Build history of the part. All positions in model axes, mm. Coordinates: 2 decimals unless noted, no trailing zeros. Order: outer loops, then holes, each group sorted by start corner. A loop starts at its lowest first (then second) coordinate and runs counter-clockwise, first axis right, second up. Notation, with made-up numbers: (87, -25) - (115, -25) arc R21 cw to (115, 7) - close; hole circle Ø6 at (81, 32.25). An arc over 180 degrees is marked (long way). Answer as CSV lines item,"result". Start each with the question number.
from build123d import *

# Parameters (mm, degrees)
SKETCH2_R               = 1.5875
SKETCH3_W               = 36.037797304
SKETCH3_H               = 47.625
CUT_EXTRUDE1_DEPTH      = 2.5875001
CUT_EXTRUDE1_DEPTH_BACK = 2.5875001


with BuildPart() as part:
    # Sweep1: sweep along a path in Sketch1
    with BuildLine(Plane.XY) as sweep1_path:
        Line((-17.4625, 889), (-17.4625, 0))
        ThreePointArc((-17.4625, 0), (0, -17.4625), (17.4625, 0))
        Line((17.4625, 0), (17.4625, 889))
        ThreePointArc((17.4625, 889), (0, 906.4625), (-17.4625, 889))
    # Sketch2 → Sweep1 (sweep)
    with BuildSketch(Plane(origin=(0, 0, 0), x_dir=(0, 0, -1), z_dir=(1, 0, 0))):
        with Locations((0, 906.4625)):
            Circle(SKETCH2_R)
    sweep(path=sweep1_path.line)

    # Sketch3 → Cut-Extrude1 (cut, two sides)
    with BuildSketch(Plane.XY) as cut_extrude1_sk:
        with Locations((-20.239587833, 623.8875)):
            Rectangle(SKETCH3_W, SKETCH3_H)
    extrude(amount=CUT_EXTRUDE1_DEPTH, mode=Mode.SUBTRACT)
    extrude(cut_extrude1_sk.sketch, amount=-CUT_EXTRUDE1_DEPTH_BACK, mode=Mode.SUBTRACT)


solid = part.part
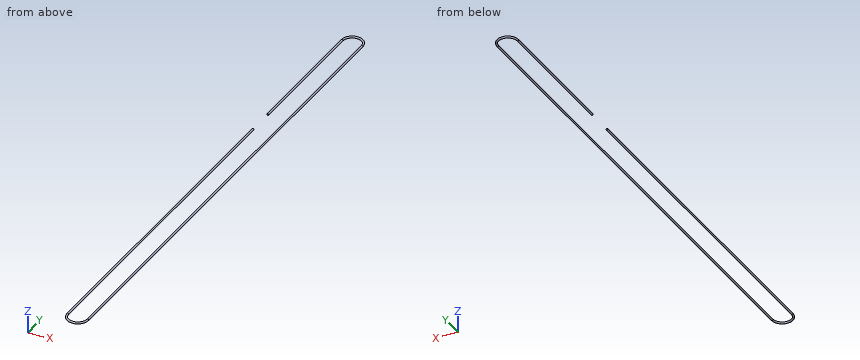
(1) Band-saw the part on B-B on y = 459. List the corners of the cut face in (x, z) (1 decimal).
(2) Probe L1, parallel to X at y = 152, z = 0.45; L2, parallel to X at y = 320.5, z = -0.6; L3, parallel to Y at x = 3, z = -1.35. List the from-to ranges inside material, lowest first. Write a range as [from, to].
(3) Band-saw the part on A-A on z = 0. List the corners of the cut face in (x, y) (3 decimals), plus the area to 3 significant figures.
(4) Drop flat-ended pins along their axis: pin 1 Ø1.6 at (x, z) = (-17, 0) entering from +Y; pin 2 Ø1 at (x, z) = (6.5, 0.5) entering from +Y; pin 3 Ø8 at (x, y) = (-9.5, 220) entering from -Z. Give the stop position or say it passes through.
Filled in:
1,outline,"circle Ø3.2 at (-17.5, 0); circle Ø3.2 at (17.5, 0)"
2,L1,"x = [-18.98, -15.94], [15.94, 18.98]"
2,L2,"x = [-18.93, -15.99], [15.99, 18.93]"
2,L3,"y = [-18.05, -16.35], [905.35, 907.05]"
3,outline,"(-19.05, 0) arc R19.05 ccw to (19.05, 0) - (19.05, 889) arc R19.05 ccw to (-19.05, 889) - (-19.05, 647.7) - (-15.875, 647.7) - (-15.875, 889) arc R15.875 cw to (15.875, 889) - (15.875, 0) arc R15.875 cw to (-15.875, 0) - (-15.875, 600.075) - (-19.05, 600.075) - close"
3,area,"5,840 mm^2"
4,pin 1,"stops at y = 899.02"
4,pin 2,"stops at y = 907.04"
4,pin 3,"passes through"
